from build123d import *

# Parameters (mm, degrees)
BOSS_EXTRUDE1_DEPTH   = 31.75
BOSS_EXTRUDE1_2_DEPTH = 31.75
BOSS_EXTRUDE1_3_DEPTH = 31.75
BOSS_EXTRUDE1_4_DEPTH = 31.75
BOSS_EXTRUDE1_5_DEPTH = 31.75
BOSS_EXTRUDE1_6_DEPTH = 31.75
BOSS_EXTRUDE1_7_DEPTH = 31.75
SKETCH2_W             = 1.5875
SKETCH2_H             = 30.1625
CUT_EXTRUDE1_DEPTH    = 166.1
SKETCH4_W             = 1.5875
SKETCH4_H             = 14.2875
BOSS_EXTRUDE2_DEPTH   = 165.1


with BuildPart() as part:
    # Sketch1 → Boss-Extrude1 (new body)
    with BuildSketch(Plane(origin=(0, 0, 0), x_dir=(1, 0, 0), z_dir=(0, 1, 0))):
        Polygon((0, 0), (0, 152.4), (12.7, 152.4), (12.7, 49.2125), (22.225, 49.2125), (22.225, 0), align=None)
    extrude(amount=BOSS_EXTRUDE1_DEPTH)


with BuildPart() as body_2:
    # Sketch1 → Boss-Extrude1 2 (new body)
    with BuildSketch(Plane(origin=(0, 0, 0), x_dir=(1, 0, 0), z_dir=(0, 1, 0))):
        Polygon((23.8125, 49.2125), (26.9875, 49.2125), (26.9875, 152.4), (42.8625, 152.4), (42.8625, 49.2125), (46.0375, 49.2125), (46.0375, 0), (23.8125, 0), align=None)
    extrude(amount=BOSS_EXTRUDE1_2_DEPTH)


with BuildPart() as body_3:
    # Sketch1 → Boss-Extrude1 3 (new body)
    with BuildSketch(Plane(origin=(0, 0, 0), x_dir=(1, 0, 0), z_dir=(0, 1, 0))):
        Polygon((47.625, 49.2125), (57.15, 49.2125), (57.15, 152.4), (69.85, 152.4), (69.85, 0), (47.625, 0), align=None)
    extrude(amount=BOSS_EXTRUDE1_3_DEPTH)


with BuildPart() as body_4:
    # Sketch1 → Boss-Extrude1 4 (new body)
    with BuildSketch(Plane(origin=(0, 0, 0), x_dir=(1, 0, 0), z_dir=(0, 1, 0))):
        Polygon((71.4375, 152.4), (71.4375, 0), (93.6625, 0), (93.6625, 49.2125), (84.1375, 49.2125), (84.1375, 152.4), align=None)
    extrude(amount=BOSS_EXTRUDE1_4_DEPTH)


with BuildPart() as body_5:
    # Sketch1 → Boss-Extrude1 5 (new body)
    with BuildSketch(Plane(origin=(0, 0, 0), x_dir=(1, 0, 0), z_dir=(0, 1, 0))):
        Polygon((95.25, 0), (95.25, 49.2125), (98.425, 49.2125), (98.425, 152.4), (111.125, 152.4), (111.125, 49.2125), (117.475, 49.2125), (117.475, 0), align=None)
    extrude(amount=BOSS_EXTRUDE1_5_DEPTH)


with BuildPart() as body_6:
    # Sketch1 → Boss-Extrude1 6 (new body)
    with BuildSketch(Plane(origin=(0, 0, 0), x_dir=(1, 0, 0), z_dir=(0, 1, 0))):
        Polygon((119.0625, 49.2125), (125.4125, 49.2125), (125.4125, 152.4), (138.1125, 152.4), (138.1125, 49.2125), (141.2875, 49.2125), (141.2875, 0), (119.0625, 0), align=None)
    extrude(amount=BOSS_EXTRUDE1_6_DEPTH)


with BuildPart() as body_7:
    # Sketch1 → Boss-Extrude1 7 (new body)
    with BuildSketch(Plane(origin=(0, 0, 0), x_dir=(1, 0, 0), z_dir=(0, 1, 0))):
        Polygon((142.875, 49.2125), (152.4, 49.2125), (152.4, 152.4), (165.1, 152.4), (165.1, 0), (142.875, 0), align=None)
    extrude(amount=BOSS_EXTRUDE1_7_DEPTH)


with BuildPart() as cut_extrude1_tool:
    # Sketch2 → Cut-Extrude1 (new body, through all)
    with BuildSketch(Plane.ZY):
        with Locations((-0.79375, 15.08125)):
            Rectangle(SKETCH2_W, SKETCH2_H)
    extrude(amount=-CUT_EXTRUDE1_DEPTH)


with BuildPart() as part_1:
    add(part.part)

    # Cut-Extrude1: cut by cut_extrude1_tool
    add(cut_extrude1_tool.part, mode=Mode.SUBTRACT)



with BuildPart() as body_2_1:
    add(body_2.part)

    # Cut-Extrude1: cut by cut_extrude1_tool
    add(cut_extrude1_tool.part, mode=Mode.SUBTRACT)


with BuildPart() as body_3_1:
    add(body_3.part)

    # Cut-Extrude1: cut by cut_extrude1_tool
    add(cut_extrude1_tool.part, mode=Mode.SUBTRACT)


with BuildPart() as body_4_1:
    add(body_4.part)

    # Cut-Extrude1: cut by cut_extrude1_tool
    add(cut_extrude1_tool.part, mode=Mode.SUBTRACT)


with BuildPart() as body_5_1:
    add(body_5.part)

    # Cut-Extrude1: cut by cut_extrude1_tool
    add(cut_extrude1_tool.part, mode=Mode.SUBTRACT)


with BuildPart() as body_6_1:
    add(body_6.part)

    # Cut-Extrude1: cut by cut_extrude1_tool
    add(cut_extrude1_tool.part, mode=Mode.SUBTRACT)


with BuildPart() as body_7_1:
    add(body_7.part)

    # Cut-Extrude1: cut by cut_extrude1_tool
    add(cut_extrude1_tool.part, mode=Mode.SUBTRACT)


with BuildPart() as part_2:
    add(part_1.part)

    add(body_2_1.part)  # Boss-Extrude2 merges body 2

    add(body_3_1.part)  # Boss-Extrude2 merges body 3

    add(body_4_1.part)  # Boss-Extrude2 merges body 4

    add(body_5_1.part)  # Boss-Extrude2 merges body 5

    add(body_6_1.part)  # Boss-Extrude2 merges body 6

    add(body_7_1.part)  # Boss-Extrude2 merges body 7
    # Sketch4 → Boss-Extrude2 (add, through all)
    with BuildSketch(Plane(origin=(0, 0, 0), x_dir=(0, 0, -1), z_dir=(1, 0, 0))):
        with Locations((153.19375, 7.14375)):
            Rectangle(SKETCH4_W, SKETCH4_H)
    extrude(amount=BOSS_EXTRUDE2_DEPTH)


solid = part_2.part
Could you check a few things on this model? Use its own coordinates, in mm. A direction names the side the tool comes from. Give positions to 0.01 mm unless a question says otherwise; leave off trailing zeros. Order: outer loops, then holes, each group sorted by start corner. A loop starts at its lowest first (then second) coordinate and runs counter-clockwise, first axis right, second up. Notation, with made-up numbers: (36, 40.5) - (90, 40.5) arc R33 cw to (90, 69.5) - close; hole circle Ø6 at (65, 86). An arc over 180 degrees is marked (long way). One line per item, written item: value. Start each with the question number.
1. For P1, Ø15.5, axis at x = 48, y = 7, coming from the +Z side; P2, Ø1.7, axis at x = 129.5, z = -0.5, coming from the -Y side; P3, Ø7.5, axis at x = 17, y = 17, coming from the -Z side; P4, Ø1.5, axis at x = 125.5, y = 17, coming from the -Z side, each with a flat end and sliding along its axis, tell me the tip position at first contact or that it passes through.
2. Imagine slicing it at B-B on x = 90. List the corners of the cut face in (y, z) for me.
3. If I drill on probe 1 along Z at (x, y) = (55, 5.5); probe 2 along Z at (x, y) = (66, 9.5); probe 3 along Z at (x, y) = (133, 29), over which ranges is the centre line in solid material (lowest first)?
4. For faces 1 (the face through (159, 23, -152.4)), 2 (the face through (35, 15, -1.588)), 3 (the face through (141.288, 16, -25)), 4 (the face through (12.7, 16, -102)), which set-ups out of +Z, -Z, +X, -X, +Y, -Y let a thin tool reach every point of the face, with its end or its side?
5. Imagine slicing it at A-A on z = -140.5. Give the number of separate pieces and of enclosed holes in the cut face, plus the area to 3 significant figures.
6. Thinking about a two-plate mould opening in X: for faces 5 (the face through (0, 16, -76)), 6 (the face through (35, 23, -152.4)), 7 (the face through (114, 16, -49.212)), which applies, +X half, -X half, draft (parallel to the pull), parting line (faces both ways), or undercut?
Values:
1. P1: z = -1.59
1. P2: y = 30.16
1. P3: z = -153.99
1. P4: z = -152.4
2. outline: (0, -153.99) - (14.29, -153.99) - (14.29, -152.4) - (0, -152.4) - close; (0, -49.21) - (31.75, -49.21) - (31.75, 0) - (30.16, 0) - (30.16, -1.59) - (0, -1.59) - close
3. probe 1: -153.99 to -152.4, -49.21 to -1.59
3. probe 2: -153.99 to -1.59
3. probe 3: -152.4 to -1.59
4. face 1: -Z, +X, -X, +Y
4. face 2: +Z, +X, -X, -Y
4. face 3: +Z, +Y, -Y
4. face 4: +Y, -Y
5. separate pieces: 7
5. enclosed holes: 0
5. area: 2,920 mm²
6. face 5: -X half
6. face 6: draft
6. face 7: undercut
